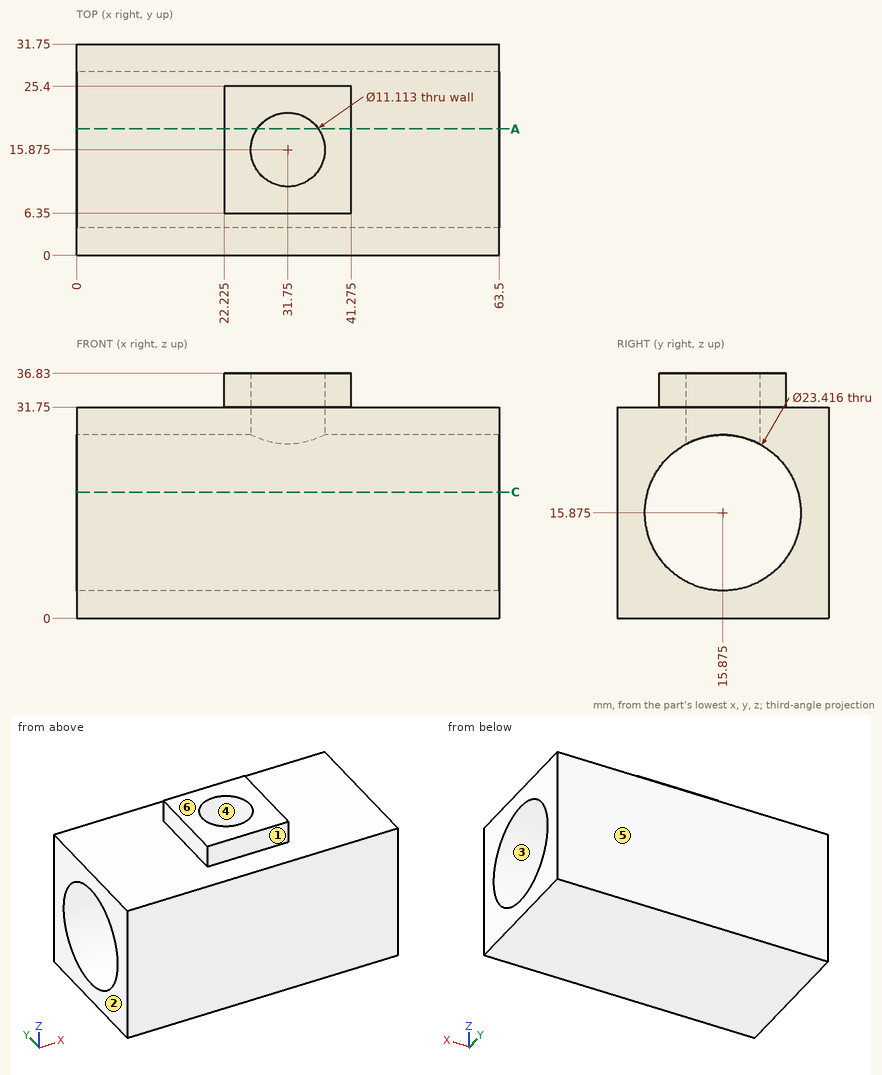
Study the drawing (mm; zero at the part's minimum x, y, z) and answer. A direction names the side the tool comes from. Coordinates: 2 decimals unless noted, no trailing zeros. Loops run counter-clockwise (first coordinate to the right, second up) from the corner with the lowest first, then second, coordinate; pieces in that order, holes last. Notation, with made-up numbers: (56.5, 8.25) -> (104.5, 8.25) arc R15 ccw to (104.5, 16.25) -> close; hole circle Ø10 at (43.5, 43.5). An arc over 180 degrees is marked (long way). Write item = value, one per line. Start each with the question number.
1) The mould has two halves that part along Y. Classify the marked faces 3, 4, 5 and 6: pulls with the +Y half, pulls with the -Y half, needs draft (parallel to the pull), parting line crosses it, or undercut.
2) For the marked faces 1 and 2, determine the directions among +Z, -Z, +X, -X, +Y, -Y from which every point of the face is accessible in a straight line to the end or side of a thin tool.
3) The part is cut by section A-A, the plane y = 19. State how many separate pieces and enclosed holes the cut face has, plus the area to 3 significant figures.
4) Find the intervals of material crossed by L1, parallel to Y at x = 31.75, z = 34.75; L2, parallel to Y at x = 11.5, z = 15.5, in increasing order. Write a range as from..to.
5) The part is cut by section C-C, the plane z = 19. Determine the outline of the cut face in (x, y), plus the area to 3 significant figures.
6) Given P1, Ø10, axis at x = 31.75, y = 15.875, coming from the +Z side; P2, Ø2, axis at x = 29, z = 24, coming from the -Y side; P3, Ø5, axis at x = 57, y = 27.5, coming from the +Z side; P4, Ø1.5, axis at x = 35, z = 35, coming from the -Y side, each flat-ended and moving along its own axis, determine where each tip first touches the part or whether it passes through.
Result:
q1.face_3 = undercut
q1.face_4 = undercut
q1.face_5 = pulls with the +Y half
q1.face_6 = needs draft
q2.face_1 = +Z, +X, -X, -Y
q2.face_2 = +Z, -Z, -X, +Y, -Y
q3.separate_pieces = 3
q3.enclosed_holes = 0
q3.area = 591 mm²
q4.L1 = 6.35..10.32, 21.43..25.4
q4.L2 = 0..4.17, 27.58..31.75
q5.outline = (0, 0) -> (63.5, 0) -> (63.5, 4.59) -> (0, 4.59) -> close; (0, 27.16) -> (63.5, 27.16) -> (63.5, 31.75) -> (0, 31.75) -> close
q5.area = 583 mm²
q6.P1 = 5.29
q6.P2 = 0
q6.P3 = 31.75
q6.P4 = 6.35
